Autodesk Inventor part; units mm, degrees
ref_plane "YZ Plane" through (0, 0, 0) normal (1, 0, 0) x (0, 1, 0)
ref_plane "XZ Plane" through (0, 0, 0) normal (0, 1, 0) x (-1, 0, 0)
ref_plane "XY Plane" through (0, 0, 0) normal (0, 0, 1) x (1, 0, 0)
sketch "Sketch1" plane through (0, 0, 0) normal (0, 0, 1) x (1, 0, 0)
  line L0 (-50.0439, 16.51) -> (-63.5, 16.51)
  line L1 (-76.2, 3.81) -> (-76.2, -3.81)
  line L2 (-76.2, -16.51) -> (76.2, 16.51) construction
  line L3 (76.2, -16.51) -> (-76.2, 16.51) construction
  line L4 (-52.2524, 10.1244) -> (-46.3865, -0.0356)
  line L5 (-46.3865, -0.0356) -> (-52.2524, -10.1956)
  line L6 (-52.2524, -10.1956) -> (-63.9841, -10.1956)
  line L7 (-63.9841, -10.1956) -> (-69.85, -0.0356)
  line L8 (-69.85, -0.0356) -> (-63.9841, 10.1244)
  line L9 (-63.9841, 10.1244) -> (-52.2524, 10.1244)
  line L10 (76.2009, -10.1956) -> (76.2, -10.1972)
  line L11 (74.477, -10.1972) -> (64.4682, -10.1972)
  line L12 (64.4682, -10.1972) -> (58.6024, -0.0372)
  line L13 (58.6024, -0.0372) -> (64.4682, 10.1228)
  line L14 (64.4682, 10.1228) -> (74.5199, 10.1228)
  line L15 (-25.4, -6.35) -> (25.4, -6.35) construction
  line L16 (25.4, -6.35) -> (25.4, 6.35) construction
  line L17 (25.4, 6.35) -> (-25.4, 6.35) construction
  line L18 (-25.4, 6.35) -> (-25.4, -6.35) construction
  line L19 (-25.4, -6.35) -> (25.4, 6.35) construction
  line L20 (25.4, -6.35) -> (-25.4, 6.35) construction
  line L21 (-44.45, 16.51) -> (-44.45, -16.51) construction
  line L22 (44.45, 16.51) -> (44.45, -16.51) construction
  arc A0 (-41.3977, 13.1123) -> (-25.4, 6.35) centre (-24.1053, 31.717) ccw
  arc A1 (-25.4, -6.35) -> (-41.3977, -13.1123) centre (-24.1053, -31.717) ccw
  arc A2 (25.4, 6.35) -> (41.3977, 13.1123) centre (24.1053, 31.717) ccw
  arc A3 (41.3977, -13.1123) -> (25.4, -6.35) centre (24.1053, -31.717) ccw
  line L23 (-25.4, 6.35) -> (25.4, 6.35)
  line L24 (-25.4, -6.35) -> (25.4, -6.35)
  arc A4 (-41.3977, 13.1123) -> (-50.0439, 16.51) centre (-50.0439, 3.81) ccw
  line L25 (-63.5, -16.51) -> (-50.0439, -16.51)
  line L26 (50.0439, -16.51) -> (63.5, -16.51)
  arc A5 (-50.0439, -16.51) -> (-41.3977, -13.1123) centre (-50.0439, -3.81) ccw
  arc A6 (41.3977, -13.1123) -> (50.0439, -16.51) centre (50.0439, -3.81) ccw
  line L27 (50.0439, 16.51) -> (63.5, 16.51)
  arc A7 (50.0439, 16.51) -> (41.3977, 13.1123) centre (50.0439, 3.81) ccw
  arc A8 (41.3977, -13.1123) -> (50.0439, -16.51) centre (50.0439, -3.81) ccw
  arc A9 (-63.5, 16.51) -> (-76.2, 3.81) centre (-63.5, 3.81) ccw
  arc A10 (-76.2, -3.81) -> (-63.5, -16.51) centre (-63.5, -3.81) ccw
  arc A11 (63.5, -16.51) -> (74.477, -10.1972) centre (63.5, -3.81) ccw
  arc A12 (74.5199, 10.1228) -> (63.5, 16.51) centre (63.5, 3.81) ccw
  line L28 (76.2, -10.1972) -> (76.2, -10.1956) construction
  line L29 (76.2, -10.1956) -> (76.2, -10.1972)
  point P0 (0, 0)
  point P1 (-58.1182, -0.0356)
  point P2 (70.3341, -0.0372)
  point P3 (76.2, 6.35)
  point P4 (41.3977, -13.1123)
  point P5 (50.0439, -16.51)
  dimension "totalLength" = 152.4
  dimension "maxWidth" = 33.02
  dimension "boltWidth" = 20.32
  dimension "d3" = 6.35
  dimension "d4" = 20.32
  dimension "handleLength" = 50.8
  dimension "handleWidth" = 12.7
  dimension "endOfHandle" = 44.45
  dimension "d8" = 44.45
  dimension "arcRadius" = 25.4
  dimension "d10" = 25.4
  dimension "d11" = 25.4
  dimension "outerFillet" = 12.7
  dimension "d15" = 12.7
  dimension "d16" = 12.7
  dimension "d17" = 12.7
extrude "Extrusion1" add sketch "Sketch1" along normal blind 6.35
equation "\"maxWidth\" = boltWidth + 2 * minWallThickness"
equation "\"boltWidth\" = boltSize + boltGap"
equation "\"d3\" = minWallThickness"
equation "\"d4\" = boltWidth"
equation "\"d15\" = outerFillet"
equation "\"d16\" = outerFillet"
equation "\"d17\" = outerFillet"
equation "\"d18\" = minWallThickness"
equation "\"minWallThickness\" = 6.35"
equation "\"boltGap\" = 1.27"
equation "\"boltSize\" = 19.05"
properties part number "3_4_inchWrenchV01"
Could you check a few things on this model? Use its own coordinates, in mm. A direction names the side the tool comes from. Coordinates: 2 decimals unless noted, no trailing zeros. Write each loop counter-clockwise with the first axis right and the second up, starting at its lowest first coordinate (ties: lowest second). Pieces come first, ordered by that corner, then holes. Notation, with made-up numbers: (82, 59.5) -> (87, 59.5) arc R8 cw to (87, 71.5) -> close; hole circle Ø1 at (61.25, 48). An arc over 180 degrees is marked (long way). One line per question, with ' | ' between items. Start each with the question number.
1. If we section it at D-D (x = 16.5): Please give me the cut outline in (y, z).
2. Thinking about a two-plate mould opening in X: for faces 6 (the face through (69.912, -14.773, 3.131)), 7 (the face through (0, -6.35, 3)), 8 (the face through (70, -10.197, 3)), which applies, pulls with the +X half, pulls with the -X half, needs draft (parallel to the pull), parting line crosses it, or undercut?
3. If we section it at C-C (y = 11.5): Please give me the cut outline in (x, z), and give its area (3 significant figures).
4. If we section it at B-B (x = -58): Please give me the cut outline in (y, z), and give its area (3 significant figures).
5. Will these pins go through, and if not, where does the flat tip stop? P1, Ø1, axis at y = -12.5, z = 3, coming from the -X side; P2, Ø1.9, axis at x = -3, z = 2, coming from the +Y side; P3, Ø3, axis at y = 7, z = 2, coming from the -X side.
6. For faces 1 (the face through (-2, 0, 6.35)), 2 (the face through (0, 6.35, 3)), 3 (the face through (33.88, -8.273, 3.131)), 4 (the face through (-58, -10.196, 3)), 5 (the face through (61.494, 4.972, 3.131)), which set-ups out of +Z, -Z, +X, -X, +Y, -Y let a thin tool reach every point of the face, with its end or its side?
7. Please list where these lines run through material, in increasing order: line 1 along Y through (x, z) = (-56, 6); line 2 along X through (y, z) = (0, 3.25); line 3 along X through (y, z) = (9, 1.5).
Return value:
1) outline: (-6.35, 0) -> (6.35, 0) -> (6.35, 6.35) -> (-6.35, 6.35) -> close
2) face 6: pulls with the +X half | face 7: undercut | face 8: needs draft
3) outline: (-73.61, 0) -> (-39.48, 0) -> (-39.48, 6.35) -> (-73.61, 6.35) -> close; (39.48, 0) -> (73.61, 0) -> (73.61, 6.35) -> (39.48, 6.35) -> close | area: 433 mm²
4) outline: (-16.51, 0) -> (-10.2, 0) -> (-10.2, 6.35) -> (-16.51, 6.35) -> close; (10.12, 0) -> (16.51, 0) -> (16.51, 6.35) -> (10.12, 6.35) -> close | area: 80.6 mm²
5) P1: stops at x = -73.21 | P2: stops at y = 6.35 | P3: stops at x = -76.09
6) face 1: +Z, +X, -X, +Y, -Y | face 2: +Z, -Z, +Y | face 3: +Z, -Z, -Y | face 4: +Z, -Z | face 5: +Z, -Z, +X
7) line 1: y = -16.51 to -10.2, 10.12 to 16.51 | line 2: x = -76.2 to -69.83, -46.41 to 58.62 | line 3: x = -75.09 to -64.63, -51.6 to -35.47, 35.47 to 63.82
